from build123d import *

# Parameters (mm, degrees)
SKETCH7_W           = 15
SKETCH7_H           = 7.5
BOSS_EXTRUDE2_DEPTH = 2
SKETCH8_R           = 1.5
BOSS_EXTRUDE3_DEPTH = 4.5
SKETCH9_R           = 1.5
CUT_EXTRUDE1_DEPTH  = 3


with BuildPart() as part:
    # Sketch7 → Boss-Extrude2 (new body)
    with BuildSketch(Plane(origin=(0, 0, 0), x_dir=(1, 0, 0), z_dir=(0, 1, 0))):
        with Locations((0, -3.75)):
            Rectangle(SKETCH7_W, SKETCH7_H)
    boss_extrude2 = extrude(amount=BOSS_EXTRUDE2_DEPTH)

    # Sketch8 → Boss-Extrude3 (add)
    with BuildSketch(Plane(origin=(0, 0, 0), x_dir=(-1, 0, 0), z_dir=(0, 0, -1))):
        with BuildLine():
            Line((-4.598991345, 11.961957852), (-7.5, 2))
            Line((-7.5, 2), (7.5, 2))
            Line((7.5, 2), (4.615024569, 11.923940807))
            ThreePointArc((4.615024569, 11.923940807), (0.020629833, 14.999957441), (-4.598991345, 11.961957852))
        make_face()
        with Locations((0, 10)):
            Circle(SKETCH8_R, mode=Mode.SUBTRACT)
    boss_extrude3 = extrude(amount=-BOSS_EXTRUDE3_DEPTH)

    # Mirror1: Boss-Extrude2, Boss-Extrude3 across plane
    add(boss_extrude2.mirror(Plane(origin=(7.5, 2, 7.5), x_dir=(1, 0, 0), z_dir=(0, 0, -1))))
    add(boss_extrude3.mirror(Plane(origin=(7.5, 2, 7.5), x_dir=(1, 0, 0), z_dir=(0, 0, -1))))

    # Sketch9 → Cut-Extrude1 (cut, through all)
    with BuildSketch(Plane(origin=(0, 2, 0), x_dir=(1, 0, 0), z_dir=(0, 1, 0))):
        with Locations((4, -7.5)):
            Circle(SKETCH9_R)
    cut_extrude1 = extrude(amount=-CUT_EXTRUDE1_DEPTH, mode=Mode.SUBTRACT)

    # Mirror2: Cut-Extrude1 across plane
    add(cut_extrude1.mirror(Plane(origin=(0, 0, 0), x_dir=(0, 0, 1), z_dir=(1, 0, 0))), mode=Mode.SUBTRACT)


solid = part.part
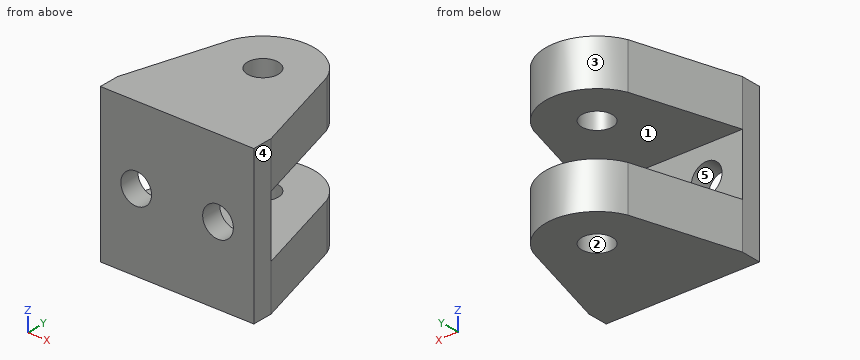
Check sheet for the modelled part. Datum: model origin and axes. Units: mm. Face numbers are marked on the shaded views. A direction names the side the tool comes from. Coordinates: 2 decimals unless noted, no trailing zeros. Write each loop counter-clockwise with the first axis right and the second up, starting at its lowest first coordinate (ties: lowest second). Pieces come first, ordered by that corner, then holes.
Item 1: Depth check by flat-ended pin: pin 1 Ø1.5 at (x, y) = (2, 5.5) entering from -Z; pin 2 Ø2.5 at (x, y) = (0, 10) entering from +Z; pin 3 Ø5 at (y, z) = (5, 2) entering from +X. Enter the tip coordinate at first touch or a pass-through.
Numbers:
pin 1: stops at z = 0
pin 2: passes through
pin 3: stops at x = 7.35
Item 2: Cross-section at B-B on x = -4. Record the boundary of the cut face in (y, z), then the cut area to 3 significant figures.
Numbers:
outline: (0, 0) - (13, 0) - (13, 4.5) - (2, 4.5) - (2, 6) - (0, 6) - close; (0, 9) - (2, 9) - (2, 10.5) - (13, 10.5) - (13, 15) - (0, 15) - close
area: 123 mm2
Item 3: Cross-section at D-D on z = 13.75. Record the boundary of the cut face in (x, y).
Numbers:
outline: (-7.5, 0) - (7.5, 0) - (7.5, 2) - (4.6, 11.96) arc R5 ccw to (-4.62, 11.92) - (-7.5, 2) - close; hole circle Ø3 at (0, 10)
Item 4: Access from +Z, -Z, +X, -X, +Y, -Y to the whole of each face (thin tool, end or side, straight path). Record for the marked faces 1 and 2.
Numbers:
face 1: +X, -X, +Y
face 2: +Z, -Z
Item 5: Mould release check, pull along X, two halves, no side actions. Record for the marked faces 3, 4 and 5: released by +X, released by -X, zero draft, split by the parting line, or undercut.
Numbers:
face 3: split by the parting line
face 4: released by +X
face 5: undercut
Item 6: Scan lines: probe 1 along X at (y, z) = (1.55, 7.5); probe 2 along Y at (x, z) = (0, 12.8); probe 3 along Z at (x, y) = (-0.75, 8.5). Record each from-to range of solid material in increasing order.
Numbers:
probe 1: x = -7.5 to -5.5, -2.5 to 2.5, 5.5 to 7.5
probe 2: y = 0 to 8.5, 11.5 to 15
probe 3: z = 0 to 4.5, 10.5 to 15
Item 7: Cross-section at A-A on z = 7.5. Record the boundary of the cut face in (x, y), then the cut area to 3 significant figures.
Numbers:
outline: (-7.5, 0) - (-5.5, 0) - (-5.5, 2) - (-7.5, 2) - close; (-2.5, 0) - (2.5, 0) - (2.5, 2) - (-2.5, 2) - close; (5.5, 0) - (7.5, 0) - (7.5, 2) - (5.5, 2) - close
area: 18.0 mm2
Item 8: Cross-section at C-C on x = 0. Record the boundary of the cut face in (y, z).
Numbers:
outline: (0, 0) - (8.5, 0) - (8.5, 4.5) - (2, 4.5) - (2, 10.5) - (8.5, 10.5) - (8.5, 15) - (0, 15) - close; (11.5, 0) - (15, 0) - (15, 4.5) - (11.5, 4.5) - close; (11.5, 10.5) - (15, 10.5) - (15, 15) - (11.5, 15) - close
